Autodesk Fusion 360 part; units mm, degrees
sketch "スケッチ1" plane through (0, 0, 0) normal (0, 0, 1) x (1, 0, 0)
  spline S0 degree 3 poles (61.2138, -44.8309) (61.2138, -44.2739) (60.7548, -43.8149) (60.1978, -43.8149) knots 0 0 0 0 1 1 1 1
  line L0 (147.3196, -135.6356) -> (137.7946, -135.6356)
  spline S1 degree 3 poles (137.0326, -134.8736) (137.0326, -135.2916) (137.3766, -135.6356) (137.7946, -135.6356) knots 0 0 0 0 1 1 1 1
  line L1 (47.8149, -147.9546) -> (282.0642, -147.9546)
  line L2 (61.2138, -52.9589) -> (74.1678, -52.9589)
  spline S2 degree 3 poles (75.4378, -43.8149) (74.7408, -43.8149) (74.1678, -44.3879) (74.1678, -45.0849) knots 0 0 0 0 1 1 1 1
  spline S3 degree 3 poles (148.2086, -131.4446) (148.2086, -131.0266) (147.8646, -130.6826) (147.4466, -130.6826) knots 0 0 0 0 1 1 1 1
  spline S4 degree 3 poles (47.8149, -43.8149) (45.6209, -43.8149) (43.8149, -45.6209) (43.8149, -47.8149) knots 0 0 0 0 1 1 1 1
  spline S5 degree 3 poles (137.5406, -130.6826) (137.2616, -130.6826) (137.0326, -130.9116) (137.0326, -131.1906) knots 0 0 0 0 1 1 1 1
  line L3 (148.2086, -131.4446) -> (148.2086, -134.7466)
  spline S6 degree 3 poles (286.0642, -47.8149) (286.0642, -45.6209) (284.2582, -43.8149) (282.0642, -43.8149) knots 0 0 0 0 1 1 1 1
  line L4 (74.1678, -52.9589) -> (74.1678, -45.0849)
  line L5 (43.8149, -143.9546) -> (43.8149, -47.8149)
  spline S7 degree 3 poles (147.3196, -135.6356) (147.8076, -135.6356) (148.2086, -135.2346) (148.2086, -134.7466) knots 0 0 0 0 1 1 1 1
  spline S8 degree 3 poles (43.8149, -143.9546) (43.8149, -146.1486) (45.6209, -147.9546) (47.8149, -147.9546) knots 0 0 0 0 1 1 1 1
  line L6 (61.2138, -44.8309) -> (61.2138, -52.9589)
  line L7 (137.5406, -130.6826) -> (147.4466, -130.6826)
  line L8 (286.0642, -143.9546) -> (286.0642, -47.8149)
  line L9 (47.8149, -43.8149) -> (60.1978, -43.8149)
  spline S9 degree 3 poles (282.0642, -147.9546) (284.2582, -147.9546) (286.0642, -146.1486) (286.0642, -143.9546) knots 0 0 0 0 1 1 1 1
  line L10 (137.0326, -134.8736) -> (137.0326, -131.1906)
  line L11 (282.0642, -43.8149) -> (75.4378, -43.8149)
  circle A0 centre (47.4979, -47.6249) radius 1.15
  circle A1 centre (231.3934, -144.1446) radius 1.15
  circle A2 centre (281.8122, -47.6249) radius 1.15
  circle A3 centre (109.9817, -144.1446) radius 1.15
  circle A4 centre (47.4979, -86.2328) radius 1.15
  circle A5 centre (129.2856, -86.2328) radius 1.15
  circle A6 centre (210.1844, -86.2328) radius 1.15
  circle A7 centre (47.4979, -144.1446) radius 1.15
  circle A8 centre (281.8122, -104.5207) radius 1.15
  circle A9 centre (281.8122, -144.1446) radius 1.15
  circle A10 centre (162.4326, -47.6249) radius 1.15
  point P0 (48.6479, -47.6249)
  point P1 (232.5434, -144.1446)
  point P2 (282.9622, -47.6249)
  point P3 (111.1317, -144.1446)
  point P4 (48.6479, -86.2328)
  point P5 (130.4356, -86.2328)
  point P6 (211.3344, -86.2328)
  point P7 (48.6479, -144.1446)
  point P8 (282.9622, -104.5207)
  point P9 (282.9622, -144.1446)
  point P10 (163.5826, -47.6249)
extrude "押し出し1" add sketch "スケッチ1" along normal blind 2
The listing builds one solid part. Answer for the finished solid, in the listing's coordinates (mm). Round coordinates to 2 decimals unless told otherwise and drop trailing zeros. Order: outer loops, then holes, each group sorted by start corner. A loop starts at its lowest first (then second) coordinate and runs counter-clockwise, first axis right, second up. Notation, with made-up numbers: (51.5, 43) -> (86.5, 43) arc R26 cw to (86.5, 69) -> close; hole circle Ø3 at (-36.75, 14.5). An arc over 180 degrees is marked (long way). Write each question's results on one line, items separated by ' | '. Start each with the question number.
Q1. Straight lines are drawn through the part: probe 1 along X at (y, z) = (-144, 1.6); probe 2 along Y at (x, z) = (138, 0.25); probe 3 along X at (y, z) = (-51.5, 1.4). For each, find the intervals that lie inside material, in ascending order. Write a range as from..to.
Q2. This flat-tipped pin is pushed along its axis until it touches: pin 1 (1.8 mm diameter, centred on x = 231.39, y = -144.14, fed in from -Z). Where does it stop, or does it pass through?
Q3. Find section A-A (x = 142.5). Determine the outline of the cut face in (y, z), then the cut area to 3 significant figures.
Worked answers:
1) probe 1: x = 43.82..46.36, 48.64..108.84, 111.12..230.25, 232.53..280.67, 282.95..286.06 | probe 2: y = -147.95..-135.64, -130.68..-43.81 | probe 3: x = 43.81..61.21, 74.17..286.06
2) pin 1: passes through
3) outline: (-147.95, 0) -> (-135.64, 0) -> (-135.64, 2) -> (-147.95, 2) -> close; (-130.68, 0) -> (-43.81, 0) -> (-43.81, 2) -> (-130.68, 2) -> close | area: 198 mm2
